Geometry check sheet. Reference: the model listing, model coordinates, mm. A direction names the side the tool comes from. Give positions to 0.01 mm unless a question says otherwise; leave off trailing zeros. Write each loop counter-clockwise with the first axis right and the second up, starting at its lowest first coordinate (ties: lowest second). Pieces come first, ordered by that corner, then holes.
(1) Thickness scan on line 1 along Y through (x, z) = (-150.5, 8.5); line 2 along X through (y, z) = (155, 23.5); line 3 along Y through (x, z) = (-148.5, 27.5). Record the ranges inside material, lowest first.
(2) Cross-section at A-A (z = 24.25). Record the boundary of the cut face in (x, y), and give its area (3 significant figures).
(3) Depth check by flat-ended pin: P1, Ø9.5, axis at x = -136.62, y = 155.45, coming from the +Z side; P2, Ø11, axis at x = 88.38, y = -69.55, coming from the +Z side; P3, Ø10, axis at y = -15, z = 26.5, coming from the -X side. Enter the tip coordinate at first touch or a pass-through.
(4) Mould release check, pull along X, two halves, no side actions. Record for faces 4 (the conical face through (-137.387, -68.843, 17.021)), 5 (the flat face through (-174.119, 34, 10)), 6 (the flat face through (120.81, 30.69, 25.07)): +X half, -X half, draft (parallel to the pull), parting line (faces both ways), or undercut.
(5) Tool access check on faces 1 (the flat face through (-25.799, -112.556, 25.07)), 2 (the cylindrical face through (105.303, -91.681, 5.07)), 3 (the cylindrical face through (89.7, 149.6, 24.9)). Record the directions out of +Z, -Z, +X, -X, +Y, -Y that give a thin tool (end or side, any length) a straight path to the whole face; none if there is none.
```python
from build123d import *

# Parameters (mm, degrees)
F1_DEPTH = 30
F3_D     = 12
F3_DEPTH = 10
F3_TIP   = 3.6051637142
F4_SIZE2 = 10
F4_SIZE  = 10
F6_D     = 12
F6_DEPTH = 10
F6_TIP   = 3.6051637142


with BuildPart() as f1:
    # F0 (on Top) → F1 (new body)
    with BuildSketch(Plane.XY):
        with BuildLine():
            Line((95.8808709681, 182.3743300438), (-144.1191290319, 182.3743300438))
            ThreePointArc((-144.1191290319, 182.3743300438), (-165.3323324675, 173.5875334794), (-174.1191290319, 152.3743300438))
            Line((-174.1191290319, 152.3743300438), (-174.1191290319, -87.6256699562))
            ThreePointArc((-174.1191290319, -87.6256699562), (-165.3323324675, -108.8388733918), (-144.1191290319, -117.6256699562))
            Line((-144.1191290319, -117.6256699562), (95.8808709681, -117.6256699562))
            ThreePointArc((95.8808709681, -117.6256699562), (117.0940744037, -108.8388733918), (125.8808709681, -87.6256699562))
            Line((125.8808709681, -87.6256699562), (125.8808709681, 152.3743300438))
            ThreePointArc((125.8808709681, 152.3743300438), (117.0940744037, 173.5875334794), (95.8808709681, 182.3743300438))
        make_face()
    extrude(amount=F1_DEPTH)

    # F3
    with Locations(Plane.XY.offset(30)):
        with Locations((-136.6191290319, 155.4529928305), (88.3808709681, 155.4529928305), (-136.6191290319, -69.5470071695), (88.3808709681, -69.5470071695)):
            Hole(F3_D / 2, depth=F3_DEPTH)
            with Locations((0, 0, -(F3_DEPTH + F3_TIP / 2))):  # 118° drill point
                Cone(0, F3_D / 2, F3_TIP, mode=Mode.SUBTRACT)

    # F4
    f4_edges = [f1.edges().sort_by_distance(p)[0] for p in [
        (-165.332332, 173.587533, 30),
        (-174.119129, 32.37433, 30),
        (-165.332332, -108.838873, 30),
        (-24.119129, -117.62567, 30),
        (117.094074, -108.838873, 30),
        (125.880871, 32.37433, 30),
        (117.094074, 173.587533, 30),
        (-24.119129, 182.37433, 30),
    ]]
    chamfer(f4_edges, length=F4_SIZE, length2=F4_SIZE2)

    # F6
    with Locations(Plane(origin=(0, 0, 0), x_dir=(1, 0, 0), z_dir=(0, 0, -1))):
        with Locations((-149.1191290319, 87.6256699562), (100.8808709681, 87.6256699562), (-149.1191290319, -162.3743300438), (100.8808709681, -162.3743300438)):
            Hole(F6_D / 2, depth=F6_DEPTH)
            with Locations((0, 0, -(F6_DEPTH + F6_TIP / 2))):  # 118° drill point
                Cone(0, F6_D / 2, F6_TIP, mode=Mode.SUBTRACT)


solid = f1.part
```
Reply:
1. line 1: y = -116.94 to -93.46, -81.79 to 156.54, 168.21 to 181.69
1. line 2: x = -170.49 to -142.6, -130.64 to 82.4, 94.36 to 122.25
1. line 3: y = -109.7 to 174.44
2. outline: (-169.87, -87.63) arc R25.75 ccw to (-144.12, -113.38) - (95.88, -113.38) arc R25.75 ccw to (121.63, -87.63) - (121.63, 152.37) arc R25.75 ccw to (95.88, 178.12) - (-144.12, 178.12) arc R25.75 ccw to (-169.87, 152.37) - close; hole circle Ø12 at (-136.62, -69.55); hole circle Ø12 at (-136.62, 155.45); hole circle Ø12 at (88.38, -69.55); hole circle Ø12 at (88.38, 155.45)
2. area: 84,000 mm2
3. P1: stops at z = 19.25
3. P2: stops at z = 19.7
3. P3: stops at x = -172.62
4. face 4: undercut
4. face 5: -X half
4. face 6: +X half
5. face 1: +Z, +X, -X, -Y
5. face 2: -Z
5. face 3: +Z
